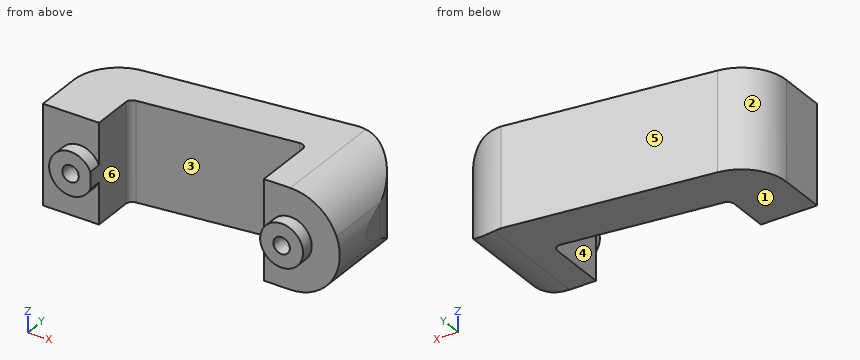
```python
from build123d import *

# Parameters (mm, degrees)
BOSS_EXTRUDE2_DEPTH = 15
CUT_EXTRUDE1_DEPTH  = 25
BOSS_EXTRUDE3_DEPTH = 10
CUT_EXTRUDE2_DEPTH  = 15
SKETCH7_R           = 3.25
SKETCH7_R_2         = 1.25
BOSS_EXTRUDE4_DEPTH = 2
SKETCH9_R           = 1.25
CUT_EXTRUDE3_DEPTH  = 10
SKETCH10_R          = 1.25
CUT_EXTRUDE4_DEPTH  = 1.5


with BuildPart() as part:
    # Sketch3 → Boss-Extrude2 (new body)
    with BuildSketch(Plane.XY):
        with BuildLine():
            Line((0, 0), (-8.5, 0))
            Line((-8.5, 0), (-8.5, 7))
            ThreePointArc((-8.5, 7), (-6.787440348, 11.510881004), (-2.512734375, 13.74869173))
            Line((-2.512734375, 13.74869173), (27.914319597, 17.399938206))
            ThreePointArc((27.914319597, 17.399938206), (33.311410485, 15.179716356), (36, 10))
            Line((36, 10), (36, 0))
            Line((36, 0), (25, 0))
            Line((25, 0), (25, 8.872825735))
            ThreePointArc((25, 8.872825735), (24.663647037, 9.620871596), (23.880854779, 9.865702574))
            Line((23.880854779, 9.865702574), (0.880854779, 7.105702574))
            ThreePointArc((0.880854779, 7.105702574), (0.251954139, 6.776472772), (0, 6.112825735))
            Line((0, 6.112825735), (0, 0))
        make_face()
    extrude(amount=BOSS_EXTRUDE2_DEPTH)

    # Sketch4 → Cut-Extrude1 (cut)
    with BuildSketch(Plane.XZ):
        with BuildLine():
            Line((36, 15), (29, 15))
            ThreePointArc((29, 15), (33.245917567, 13.68240924), (36, 10.192582404))
            Line((36, 10.192582404), (36, 15))
        make_face()
        with BuildLine():
            Line((36, 0), (36, 4.807417596))
            ThreePointArc((36, 4.807417596), (33.245917567, 1.31759076), (29, 0))
            Line((29, 0), (36, 0))
        make_face()
    extrude(amount=-CUT_EXTRUDE1_DEPTH, mode=Mode.SUBTRACT)

    # Sketch5 → Boss-Extrude3 (add)
    with BuildSketch(Plane.XZ):
        with BuildLine():
            ThreePointArc((36, 4.807417596), (36.5, 7.5), (36, 10.192582404))
            Line((36, 10.192582404), (36, 4.807417596))
        make_face()
    extrude(amount=-BOSS_EXTRUDE3_DEPTH)

    # Sketch6 → Cut-Extrude2 (cut)
    with BuildSketch(Plane.XY.offset(15)):
        Polygon((36.5, 10), (36, 10), (36.5, 6.112287873), align=None)
    extrude(amount=-CUT_EXTRUDE2_DEPTH, mode=Mode.SUBTRACT)

    # Sketch7 → Boss-Extrude4 (add)
    with BuildSketch(Plane.XZ):
        with Locations((29, 7.5)):
            Circle(SKETCH7_R)
        with Locations((29, 7.5)):
            Circle(SKETCH7_R_2, mode=Mode.SUBTRACT)
        with BuildLine():
            Line((0, 8.75), (0, 6.25))
            ThreePointArc((0, 6.25), (-6.25, 7.5), (0, 8.75))
        make_face()
        with Locations((-3, 7.5)):
            Circle(SKETCH7_R_2, mode=Mode.SUBTRACT)
    extrude(amount=BOSS_EXTRUDE4_DEPTH)

    # Sketch9 → Cut-Extrude3 (cut)
    with BuildSketch(Plane.XZ.offset(2)):
        with Locations((29, 7.5)):
            Circle(SKETCH9_R)
        with Locations((-3, 7.5)):
            Circle(SKETCH9_R)
    extrude(amount=-CUT_EXTRUDE3_DEPTH, mode=Mode.SUBTRACT)

    # Sketch10 → Cut-Extrude4 (cut)
    with BuildSketch(Plane.XZ.offset(-8)):
        with Locations((29, 7.5)):
            Circle(SKETCH10_R)
    extrude(amount=-CUT_EXTRUDE4_DEPTH, mode=Mode.SUBTRACT)


solid = part.part
```
Input: part model. Units: mm. Frame: model coordinates. Face numbers are marked on the shaded views. A direction names the side the tool comes from. Give positions to 0.01 mm unless a question says otherwise; leave off trailing zeros. Order: outer loops, then holes, each group sorted by start corner. A loop starts at its lowest first (then second) coordinate and runs counter-clockwise, first axis right, second up. Notation, with made-up numbers: (34, 24.5) - (92, 24.5) arc R18 cw to (92, 29.5) - close; hole circle Ø11 at (-1, 24). An arc over 180 degrees is marked (long way). Put each result on its own line as item: value.
Item 1: Access query for the marked faces 5 and 6. Directions: +Z, -Z, +X, -X, +Y, -Y. A direction counts if a zero-diameter tool reaches every point of the face in a straight line with its end or side. Return the directions, or none.
Found:
face 5: +Z, -Z, -X, +Y
face 6: +Z, -Z, -Y
Item 2: Section query B-B, the plane z = 7.5. Return loops of the section in (x, y).
Found:
outline: (-8.5, 0) - (-6.25, 0) - (-6.25, -2) - (-4.25, -2) - (-4.25, 8) - (-1.75, 8) - (-1.75, -2) - (0, -2) - (0, 6.11) arc R1 cw to (0.88, 7.11) - (23.88, 9.87) arc R1 cw to (25, 8.87) - (25, 0) - (25.75, 0) - (25.75, -2) - (27.75, -2) - (27.75, 9.5) - (30.25, 9.5) - (30.25, -2) - (32.25, -2) - (32.25, 0) - (36.5, 0) - (36.5, 6.11) - (36, 10) arc R8.49 ccw to (27.91, 17.4) - (-2.51, 13.75) arc R6.8 ccw to (-8.5, 7) - close
Item 3: Section query D-D, the plane y = 11.75. Return loops of the section in (x, z).
Found:
outline: (-6.56, 0) - (29, 0) arc R7.5 ccw to (35.58, 3.91) - (35.58, 11.09) arc R7.5 ccw to (29, 15) - (-6.56, 15) - close
Item 4: Ray query, L1, parallel to Z at x = -3, y = 3.5; L2, parallel to Z at x = -3, y = -1.2; L3, parallel to X at y = 2.25, z = 9. Return the intervals inside material, ascending. Write a range as from..to.
Found:
L1: z = 0..6.25, 8.75..15
L2: z = 4.25..6.25, 8.75..10.75
L3: x = -8.5..0, 25..36.35
Item 5: Section query C-C, the plane x = -3. Return loops of the section in (y, z), then the cut area to 3 significant figures.
Found:
outline: (-2, 4.25) - (0, 4.25) - (0, 0) - (13.67, 0) - (13.67, 15) - (0, 15) - (0, 10.75) - (-2, 10.75) - (-2, 8.75) - (8, 8.75) - (8, 6.25) - (-2, 6.25) - close
area: 193 mm^2
Item 6: Contact query for flat-ended pins moving along their axis: pin 1 (2 mm diameter, centred on x = 29, z = 7.5, fed in from +Y); pin 2 (2 mm diameter, centred on x = -3, z = 7.5, fed in from +Y); pin 3 (1 mm diameter, centred on x = 6.5, z = 4.5, fed in from -Y). Output: stop coordinate, or through.
Found:
pin 1: stops at y = 17.4
pin 2: stops at y = 13.81
pin 3: stops at y = 7.72
Item 7: Draft query along X for the marked faces 1, 2, 3 and 4. Return one class per face: +X half, -X half, draft (parallel to the pull), parting line (faces both ways), or undercut.
Found:
face 1: draft
face 2: -X half
face 3: undercut
face 4: undercut
Item 8: Section query A-A, the plane y = 2.5. Return loops of the section in (x, z).
Found:
outline: (-8.5, 0) - (0, 0) - (0, 15) - (-8.5, 15) - close; (25, 0) - (29, 0) arc R7.5 ccw to (29, 15) - (25, 15) - close; hole circle Ø2.5 at (-3, 7.5); hole circle Ø2.5 at (29, 7.5)
